```python
from build123d import *

# Parameters (mm, degrees)
BOSS_EXTRUDE1_DEPTH = 19
CUT_EXTRUDE1_REACH  = 40.1
SKETCH3_R           = 5.99948
CUT_EXTRUDE2_REACH  = 40.1
TOP_VIEW_R          = 1.5875


with BuildPart() as part:
    # Sketch2 → Boss-Extrude1 (new body)
    with BuildSketch(Plane.XY):
        with BuildLine():
            Line((-19.05, 0), (19.05, 0))
            Line((19.05, 0), (19.05, 38.1))
            Line((19.05, 38.1), (18.25625, 38.1))
            ThreePointArc((18.25625, 38.1), (17.694983992, 37.867516008), (17.4625, 37.30625))
            Line((17.4625, 37.30625), (17.4625, 2.38125))
            ThreePointArc((17.4625, 2.38125), (17.230016008, 1.819983992), (16.66875, 1.5875))
            Line((16.66875, 1.5875), (-18.25625, 1.5875))
            ThreePointArc((-18.25625, 1.5875), (-18.817516008, 1.355016008), (-19.05, 0.79375))
            Line((-19.05, 0.79375), (-19.05, 0))
        make_face()
    extrude(amount=-BOSS_EXTRUDE1_DEPTH)

    # Sketch3 → Cut-Extrude1 (cut, up to next)
    with BuildSketch(Plane(origin=(19.05, 0, 0), x_dir=(0, 0, -1), z_dir=(1, 0, 0)), mode=Mode.PRIVATE) as cut_extrude1_sk1:
        with Locations((9.5, 25)):
            Circle(SKETCH3_R)
    cut_extrude1_tool1 = extrude(cut_extrude1_sk1.sketch, amount=-CUT_EXTRUDE1_REACH, mode=Mode.PRIVATE) & part.part
    add(cut_extrude1_tool1.solids().sort_by_distance((19.05, 25, -9.5))[0], mode=Mode.SUBTRACT)
    # Sketch3 → Cut-Extrude1 (cut, up to next)
    with BuildSketch(Plane(origin=(19.05, 0, 0), x_dir=(0, 0, -1), z_dir=(1, 0, 0)), mode=Mode.PRIVATE) as cut_extrude1_sk2:
        with BuildLine():
            ThreePointArc((12.75, 30.629165125), (12.383974596, 31.995190528), (13.75, 32.361215932))
            ThreePointArc((13.75, 32.361215932), (14.116025404, 30.995190528), (12.75, 30.629165125))
        make_face()
    cut_extrude1_tool2 = extrude(cut_extrude1_sk2.sketch, amount=-CUT_EXTRUDE1_REACH, mode=Mode.PRIVATE) & part.part
    add(cut_extrude1_tool2.solids().sort_by_distance((19.05, 31.495191, -13.25))[0], mode=Mode.SUBTRACT)
    # Sketch3 → Cut-Extrude1 (cut, up to next)
    with BuildSketch(Plane(origin=(19.05, 0, 0), x_dir=(0, 0, -1), z_dir=(1, 0, 0)), mode=Mode.PRIVATE) as cut_extrude1_sk3:
        with BuildLine():
            ThreePointArc((12.75, 19.370834875), (14.116025404, 19.004809472), (13.75, 17.638784068))
            ThreePointArc((13.75, 17.638784068), (12.383974596, 18.004809472), (12.75, 19.370834875))
        make_face()
    cut_extrude1_tool3 = extrude(cut_extrude1_sk3.sketch, amount=-CUT_EXTRUDE1_REACH, mode=Mode.PRIVATE) & part.part
    add(cut_extrude1_tool3.solids().sort_by_distance((19.05, 18.504809, -13.25))[0], mode=Mode.SUBTRACT)
    # Sketch3 → Cut-Extrude1 (cut, up to next)
    with BuildSketch(Plane(origin=(19.05, 0, 0), x_dir=(0, 0, -1), z_dir=(1, 0, 0)), mode=Mode.PRIVATE) as cut_extrude1_sk4:
        with BuildLine():
            ThreePointArc((1, 25), (2, 26), (3, 25))
            ThreePointArc((3, 25), (2, 24), (1, 25))
        make_face()
    cut_extrude1_tool4 = extrude(cut_extrude1_sk4.sketch, amount=-CUT_EXTRUDE1_REACH, mode=Mode.PRIVATE) & part.part
    add(cut_extrude1_tool4.solids().sort_by_distance((19.05, 25, -2))[0], mode=Mode.SUBTRACT)

    # Top View → Cut-Extrude2 (cut, up to next)
    with BuildSketch(Plane.XZ, mode=Mode.PRIVATE) as cut_extrude2_sk1:
        with Locations((-12.7, -15.825)):
            Circle(TOP_VIEW_R)
    cut_extrude2_tool1 = extrude(cut_extrude2_sk1.sketch, amount=-CUT_EXTRUDE2_REACH, mode=Mode.PRIVATE) & part.part
    add(cut_extrude2_tool1.solids().sort_by_distance((-12.7, 0, -15.825))[0], mode=Mode.SUBTRACT)
    # Top View → Cut-Extrude2 (cut, up to next)
    with BuildSketch(Plane.XZ, mode=Mode.PRIVATE) as cut_extrude2_sk2:
        with Locations((12.7, -15.825)):
            Circle(TOP_VIEW_R)
    cut_extrude2_tool2 = extrude(cut_extrude2_sk2.sketch, amount=-CUT_EXTRUDE2_REACH, mode=Mode.PRIVATE) & part.part
    add(cut_extrude2_tool2.solids().sort_by_distance((12.7, 0, -15.825))[0], mode=Mode.SUBTRACT)
    # Top View → Cut-Extrude2 (cut, up to next)
    with BuildSketch(Plane.XZ, mode=Mode.PRIVATE) as cut_extrude2_sk3:
        with Locations((12.7, -3.175)):
            Circle(TOP_VIEW_R)
    cut_extrude2_tool3 = extrude(cut_extrude2_sk3.sketch, amount=-CUT_EXTRUDE2_REACH, mode=Mode.PRIVATE) & part.part
    add(cut_extrude2_tool3.solids().sort_by_distance((12.7, 0, -3.175))[0], mode=Mode.SUBTRACT)
    # Top View → Cut-Extrude2 (cut, up to next)
    with BuildSketch(Plane.XZ, mode=Mode.PRIVATE) as cut_extrude2_sk4:
        with Locations((-12.7, -3.175)):
            Circle(TOP_VIEW_R)
    cut_extrude2_tool4 = extrude(cut_extrude2_sk4.sketch, amount=-CUT_EXTRUDE2_REACH, mode=Mode.PRIVATE) & part.part
    add(cut_extrude2_tool4.solids().sort_by_distance((-12.7, 0, -3.175))[0], mode=Mode.SUBTRACT)


solid = part.part
```
The model under review builds one solid part; all positions refer to its coordinate system, in mm. A direction names the side the tool comes from. Give positions to 0.01 mm unless a question says otherwise; leave off trailing zeros. Write each loop counter-clockwise with the first axis right and the second up, starting at its lowest first coordinate (ties: lowest second). Pieces come first, ordered by that corner, then holes.
(1) Consider section A-A, the plane y = 25. Give the boundary of the cut face in (x, z), and give its area (3 significant figures).
(2) Tool access review of faces 1 (the cylindrical face through (18, 26, -2)), 2 (the flat face through (17.462, 16, -9)): name each direction out of +Z, -Z, +X, -X, +Y, -Y from which nothing blocks a thin tool from reaching the whole face with its end or side.
(3) To check wall thickness, follow L1, parallel to Z at x = -12.7, y = 1.1; L2, parallel to Z at x = -12, y = 1; L3, parallel to Y at x = 18.6, z = -2. State the ranges of each line that lie inside material, in increasing order.
(4) For P1, Ø8, axis at x = 7, z = -14.5, coming from the +Y side; P2, Ø9.5, axis at y = 26, z = -8.5, coming from the -X side, all flat-tipped, find the tip position at first contact; note any pin that passes through.
(5) Consider section B-B, the plane x = -12.7. Give the boundary of the cut face in (y, z).
(6) Consider section D-D, the plane z = -16.75. Give the boundary of the cut face in (x, y), and give its area (3 significant figures).
(7) The part is to be moulded in two halves that separate along Z. For faces 3 (the flat face through (18, 11, 0)), 4 (the cylindrical face through (-11.234, 0.783, -3.783)), 5 (the flat face through (-1, 1.588, -9)), say which applies: released by +Z, released by -Z, zero draft, split by the parting line, or undercut.
(8) Consider section C-C, the plane z = -9.5. Give the boundary of the cut face in (x, y), and give its area (3 significant figures).
Returned:
1. outline: (17.46, -19) - (19.05, -19) - (19.05, -15.5) - (17.46, -15.5) - close; (17.46, -3.5) - (19.05, -3.5) - (19.05, -3) - (17.46, -3) - close; (17.46, -1) - (19.05, -1) - (19.05, 0) - (17.46, 0) - close
1. area: 7.94 mm2
2. face 1: +X, -X
2. face 2: +Z, -Z, -X, +Y
3. L1: z = -19 to -17.41, -14.24 to -4.76, -1.59 to 0
3. L2: z = -19 to -17.25, -14.4 to -4.6, -1.75 to 0
3. L3: y = 0 to 24, 26 to 38.1
4. P1: stops at y = 1.59
4. P2: stops at x = 17.46
5. outline: (0, -19) - (1.59, -19) - (1.59, -17.41) - (0, -17.41) - close; (0, -14.24) - (1.59, -14.24) - (1.59, -4.76) - (0, -4.76) - close; (0, -1.59) - (1.59, -1.59) - (1.59, 0) - (0, 0) - close
6. outline: (-19.05, 0) - (-13.99, 0) - (-13.99, 1.59) - (-18.26, 1.59) arc R0.79 ccw to (-19.05, 0.79) - close; (-11.41, 0) - (11.41, 0) - (11.41, 1.59) - (-11.41, 1.59) - close; (13.99, 0) - (19.05, 0) - (19.05, 38.1) - (18.26, 38.1) arc R0.79 ccw to (17.46, 37.31) - (17.46, 2.38) arc R0.79 cw to (16.67, 1.59) - (13.99, 1.59) - close
6. area: 110 mm2
7. face 3: released by +Z
7. face 4: undercut
7. face 5: zero draft
8. outline: (-19.05, 0) - (19.05, 0) - (19.05, 19) - (17.46, 19) - (17.46, 2.38) arc R0.79 cw to (16.67, 1.59) - (-18.26, 1.59) arc R0.79 ccw to (-19.05, 0.79) - close; (17.46, 31) - (19.05, 31) - (19.05, 38.1) - (18.26, 38.1) arc R0.79 ccw to (17.46, 37.31) - close
8. area: 99.3 mm2
